```python
from build123d import *

# Parameters (mm, degrees)
SKETCH1_W           = 25.59
SKETCH1_H           = 10.8
SKETCH1_W_2         = 19.76
SKETCH1_H_2         = 4.8
BOSS_EXTRUDE1_DEPTH = 8
CUT_EXTRUDE3_DEPTH  = 11.8
FILLET2_R           = 2
FILLET3_R           = 2
SKETCH3_W           = 24
SKETCH3_H           = 8.8
CUT_EXTRUDE2_DEPTH  = 1
FILLET4_R           = 2


with BuildPart() as part:
    # Sketch1 → Boss-Extrude1 (new body)
    with BuildSketch(Plane(origin=(0, 0, 0), x_dir=(1, 0, 0), z_dir=(0, 1, 0))):
        Rectangle(SKETCH1_W, SKETCH1_H)
        Rectangle(SKETCH1_W_2, SKETCH1_H_2, mode=Mode.SUBTRACT)
    extrude(amount=BOSS_EXTRUDE1_DEPTH)

    # Sketch4 → Cut-Extrude3 (cut, through all)
    with BuildSketch(Plane.XY.offset(5.4)):
        with BuildLine():
            Line((-12.795, 0), (-12.795, 9.131507451))
            Line((-12.795, 9.131507451), (12.795, 9.131507451))
            Line((12.795, 9.131507451), (12.795, 0))
            add(Edge.make_bspline(
                [(-12.795, 0), (-12.426580691, 7.502461836), (0, 8.497538164), (12.426580691, 7.502461836), (12.795, 0)],
                knots=[0, 0, 0, 0, 0.5, 1, 1, 1, 1], degree=3))
        make_face()
    extrude(amount=-CUT_EXTRUDE3_DEPTH, mode=Mode.SUBTRACT)

    # Fillet2
    fillet2_edges = [part.edges().sort_by_distance(p)[0] for p in [
        (8.47733972, 6.862563229, 5.4),
        (-8.477340259, 6.862562997, 5.4),
    ]]
    fillet(fillet2_edges, radius=FILLET2_R)

    # Fillet3
    fillet3_edges = [part.edges().sort_by_distance(p)[0] for p in [
        (8.47734001, 6.862563107, -5.4),
        (-8.477339964, 6.862563119, -5.4),
    ]]
    fillet(fillet3_edges, radius=FILLET3_R)

    # Sketch3 → Cut-Extrude2 (cut)
    with BuildSketch(Plane.XZ):
        Rectangle(SKETCH3_W, SKETCH3_H)
    extrude(amount=-CUT_EXTRUDE2_DEPTH, mode=Mode.SUBTRACT)

    # Fillet4
    fillet4_edges = [part.edges().sort_by_distance(p)[0] for p in [
        (12, 0.5, 4.4),
        (12, 0.5, -4.4),
        (-12, 0.5, -4.4),
        (-12, 0.5, 4.4),
    ]]
    fillet(fillet4_edges, radius=FILLET4_R)


solid = part.part
```
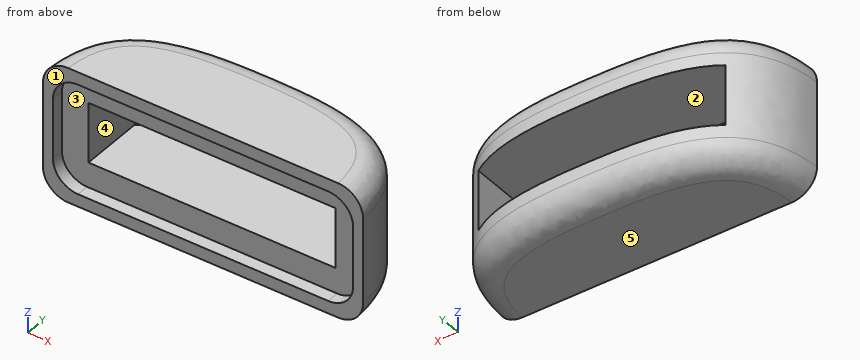
Read the model definition and answer for the solid it produces. Units are mm, in the model's axes. Face numbers are marked on the shaded views. A direction names the side the tool comes from. Round coordinates to 2 decimals unless told otherwise and drop trailing zeros. One line per item, written item: value.
Q1. For a pull along X with two mould halves and no side action, classify the marked faces 1 and 2 as +X half, -X half, draft (parallel to the pull), parting line (faces both ways), or undercut.
Data:
face 1: draft
face 2: undercut
Q2. Straight lines are drawn through the part: line 1 (Z direction, x = -4.25, y = 3.5); line 2 (Z direction, x = -8, y = 0.75); line 3 (Y direction, x = 10, z = 2.5). For each, find the intervals that lie inside material, in ascending order. Write a range as [from, to].
Data:
line 1: [-5.4, -2.4], [2.4, 5.4]
line 2: [-5.4, -4.4], [4.4, 5.4]
line 3: [1, 6]
Q3. Flat-ended cylindrical pins translate along their axes: pin 1 Ø4 at (y, z) = (3, -1) entering from +X; pin 2 Ø0.8 at (y, z) = (0.5, 0.5) entering from -X; pin 3 Ø3 at (y, z) = (5.5, -2.5) entering from +X. Find the tip coordinate at first contact, or state that the pin passes through.
Data:
pin 1: x = 12.71
pin 2: x = -12.79
pin 3: x = 11.77
Q4. Which of the six approach directions +Z, -Z, +X, -X, +Y, -Y give full straight-line access (tool end or side, diameter ignored) to the marked faces 3, 4 and 5?
Data:
face 3: -Y
face 4: +Y, -Y
face 5: -Z, +X, -X, +Y, -Y
